Input: part model. Units: mm. Frame: model coordinates. Face numbers are marked on the shaded views. Coordinates: 2 decimals unless noted, no trailing zeros. Order: outer loops, then holes, each group sorted by start corner. A loop starts at its lowest first (then second) coordinate and runs counter-clockwise, first axis right, second up. Notation, with made-up numbers: (-38.75, 60.25) -> (14.25, 60.25) arc R32 cw to (14.25, 99.25) -> close; hole circle Ø4 at (56.25, 6). An arc over 180 degrees is marked (long way). One line per question, with ' | ' between items.
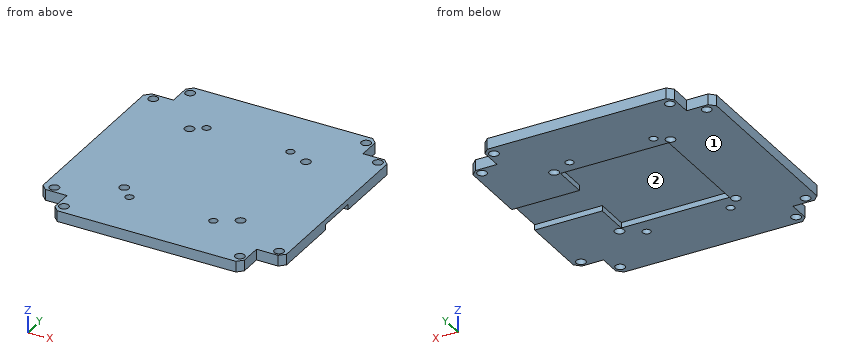
```python
from build123d import *

# Parameters (mm, degrees)
SKETCH1_W           = 90
SKETCH1_H           = 70
BOSS_EXTRUDE1_DEPTH = 4
SKETCH2_R           = 1.75
CUT_EXTRUDE1_DEPTH  = 5
CHAMFER1_SIZE       = 2
CHAMFER2_SIZE       = 2
CHAMFER3_SIZE       = 2
CHAMFER4_SIZE       = 2
SKETCH5_W           = 70
SKETCH5_H           = 4
BOSS_EXTRUDE3_DEPTH = 10
SKETCH4_W           = 70
SKETCH4_H           = 4
BOSS_EXTRUDE4_DEPTH = 10
SKETCH6_R           = 1.75
CUT_EXTRUDE2_DEPTH  = 10
CHAMFER5_SIZE       = 2
SKETCH7_W           = 40
SKETCH7_H           = 40
CUT_EXTRUDE3_DEPTH  = 2
SKETCH8_W           = 25
SKETCH8_H           = 15
CUT_EXTRUDE4_DEPTH  = 2
SKETCH9_R           = 1.5
CUT_EXTRUDE5_DEPTH  = 4


with BuildPart() as part:
    # Sketch1 → Boss-Extrude1 (new body)
    with BuildSketch(Plane.XY):
        with Locations((44.768273235, 35.193370166)):
            Rectangle(SKETCH1_W, SKETCH1_H)
    extrude(amount=BOSS_EXTRUDE1_DEPTH)

    # Sketch2 → Cut-Extrude1 (cut)
    with BuildSketch(Plane.XY.offset(4)):
        with Locations((3.703568783, 2.693370166)):
            Circle(SKETCH2_R)
        with Locations((86.703568783, 2.694436567)):
            Circle(SKETCH2_R)
        with Locations((86.703273235, 67.693370166)):
            Circle(SKETCH2_R)
        with Locations((3.703273235, 67.693370166)):
            Circle(SKETCH2_R)
        with Locations((23.297725672, 13.693370166)):
            Circle(SKETCH2_R)
        with Locations((66.284051901, 13.693370166)):
            Circle(SKETCH2_R)
        with Locations((66.268273235, 56.693370166)):
            Circle(SKETCH2_R)
        with Locations((23.268273235, 56.693370166)):
            Circle(SKETCH2_R)
    extrude(amount=-CUT_EXTRUDE1_DEPTH, mode=Mode.SUBTRACT)

    # Chamfer1
    chamfer1_edges = [part.edges().sort_by_distance(p)[0] for p in [
        (89.768273235, 0.193370166, 2),
    ]]
    chamfer(chamfer1_edges, length=CHAMFER1_SIZE)

    # Chamfer2
    chamfer2_edges = [part.edges().sort_by_distance(p)[0] for p in [
        (-0.231726765, 0.193370166, 2),
    ]]
    chamfer(chamfer2_edges, length=CHAMFER2_SIZE)

    # Chamfer3
    chamfer3_edges = [part.edges().sort_by_distance(p)[0] for p in [
        (-0.231726765, 70.193370166, 2),
    ]]
    chamfer(chamfer3_edges, length=CHAMFER3_SIZE)

    # Chamfer4
    chamfer4_edges = [part.edges().sort_by_distance(p)[0] for p in [
        (89.768273235, 70.193370166, 2),
    ]]
    chamfer(chamfer4_edges, length=CHAMFER4_SIZE)

    # Sketch5 → Boss-Extrude3 (add)
    with BuildSketch(Plane(origin=(0, 70.193370166, 0), x_dir=(1, 0, 0), z_dir=(0, 1, 0))):
        with Locations((44.768273235, -2)):
            Rectangle(SKETCH5_W, SKETCH5_H)
    extrude(amount=BOSS_EXTRUDE3_DEPTH)

    # Sketch4 → Boss-Extrude4 (add)
    with BuildSketch(Plane(origin=(0, 0.193370166, 0), x_dir=(-1, 0, 0), z_dir=(0, -1, 0))):
        with Locations((-44.768273235, -2)):
            Rectangle(SKETCH4_W, SKETCH4_H)
    extrude(amount=BOSS_EXTRUDE4_DEPTH)

    # Sketch6 → Cut-Extrude2 (cut)
    with BuildSketch(Plane(origin=(0, 0, 0), x_dir=(-1, 0, 0), z_dir=(0, 0, -1))):
        with Locations((-12.268273235, 76.693370166)):
            Circle(SKETCH6_R)
        with Locations((-77.268273235, 76.693370166)):
            Circle(SKETCH6_R)
        with Locations((-77.268273235, -6.306629834)):
            Circle(SKETCH6_R)
        with Locations((-12.268273235, -6.306629834)):
            Circle(SKETCH6_R)
    extrude(amount=-CUT_EXTRUDE2_DEPTH, mode=Mode.SUBTRACT)

    # Chamfer5
    chamfer5_edges = [part.edges().sort_by_distance(p)[0] for p in [
        (9.768273235, 80.193370166, 2),
        (79.768273235, 80.193370166, 2),
        (9.768273235, -9.806629834, 2),
        (79.768273235, -9.806629834, 2),
    ]]
    chamfer(chamfer5_edges, length=CHAMFER5_SIZE)

    # Sketch7 → Cut-Extrude3 (cut)
    with BuildSketch(Plane(origin=(0, 0, 0), x_dir=(-1, 0, 0), z_dir=(0, 0, -1))):
        with Locations((-44.768273235, 35.193370166)):
            Rectangle(SKETCH7_W, SKETCH7_H)
    extrude(amount=-CUT_EXTRUDE3_DEPTH, mode=Mode.SUBTRACT)

    # Sketch8 → Cut-Extrude4 (cut)
    with BuildSketch(Plane(origin=(0, 0, 0), x_dir=(-1, 0, 0), z_dir=(0, 0, -1))):
        with Locations((-77.268273235, 35.193370166)):
            Rectangle(SKETCH8_W, SKETCH8_H)
    extrude(amount=-CUT_EXTRUDE4_DEPTH, mode=Mode.SUBTRACT)

    # Sketch9 → Cut-Extrude5 (cut)
    with BuildSketch(Plane(origin=(0, 0, 0), x_dir=(-1, 0, 0), z_dir=(0, 0, -1))):
        with Locations((-27.768273235, 9.193370166)):
            Circle(SKETCH9_R)
        with Locations((-58.768273235, 9.193370166)):
            Circle(SKETCH9_R)
        with Locations((-27.768273235, 59.856282799)):
            Circle(SKETCH9_R)
        with Locations((-58.768273235, 59.856282799)):
            Circle(SKETCH9_R)
    extrude(amount=-CUT_EXTRUDE5_DEPTH, mode=Mode.SUBTRACT)


solid = part.part
```
1. Cut plane C-C, the plane x = 23.5. Return loops of the section in (y, z).
Recorded:
outline: (-9.81, 0) -> (11.96, 0) -> (11.96, 4) -> (-9.81, 4) -> close; (15.43, 0) -> (54.96, 0) -> (54.96, 4) -> (15.43, 4) -> close; (58.43, 0) -> (80.19, 0) -> (80.19, 4) -> (58.43, 4) -> close
2. Cut plane A-A, the plane x = 52. Return loops of the section in (y, z).
Recorded:
outline: (-9.81, 0) -> (15.19, 0) -> (15.19, 2) -> (55.19, 2) -> (55.19, 0) -> (80.19, 0) -> (80.19, 4) -> (-9.81, 4) -> close
3. Mould query, pull axis Y, two halves, no side actions, for the marked faces 1 and 2. Classes: released by +Y, released by -Y, zero draft, split by the parting line, or undercut.
Recorded:
face 1: zero draft | face 2: undercut
4. Cut plane B-B, the plane y = 39. Return loops of the section in (x, z).
Recorded:
outline: (-0.23, 0) -> (24.77, 0) -> (24.77, 2) -> (89.77, 2) -> (89.77, 4) -> (-0.23, 4) -> close
5. Pin query (flat end, axial travel): pin 1 Ø1 at (y, z) = (69, 3.5) entering from +X; pin 2 Ø1.2 at (y, z) = (-4.5, 1) entering from +X. Return the tip coordinate at first contact, or that it passes through.
Recorded:
pin 1: stops at x = 89.46 | pin 2: stops at x = 79.77
6. Ray query, line 1 (X direction, y = 2.5, z = 2); line 2 (Y direction, x = 57, z = 1.75); line 3 (Y direction, x = 11.5, z = 0.55). Return the intervals inside material, ascending. Write a range as [from, to].
Recorded:
line 1: x = [-0.23, 1.96], [5.44, 84.96], [88.44, 89.77] | line 2: y = [-9.81, 15.19], [55.19, 80.19] | line 3: y = [-9.54, -7.88], [-4.73, 75.12], [78.27, 79.93]
7. Cut plane D-D, the plane y = 53. Return loops of the section in (x, z), and give its area (3 significant figures).
Recorded:
outline: (-0.23, 0) -> (24.77, 0) -> (24.77, 2) -> (64.77, 2) -> (64.77, 0) -> (89.77, 0) -> (89.77, 4) -> (-0.23, 4) -> close | area: 280 mm^2
